The listing builds one solid part. Answer for the finished solid, in the listing's coordinates (mm). A direction names the side the tool comes from. Coordinates: 2 decimals unless noted, no trailing zeros. Order: outer loops, then holes, each group sorted by start corner. A loop starts at its lowest first (then second) coordinate and runs counter-clockwise, first axis right, second up. Notation, with made-up numbers: (49.5, 52) -> (108.5, 52) arc R32 ccw to (108.5, 85) -> close; hole circle Ø4 at (53.25, 10). An arc over 180 degrees is marked (long way). Return JSON: item names as keys, results as strings.
```python
from build123d import *

# Parameters (mm, degrees)
SKETCH1_W           = 50
SKETCH1_H           = 50
BOSS_EXTRUDE1_DEPTH = 25
SHELL1_T            = -2
SKETCH3_W           = 10
SKETCH3_H           = 6
CUT_EXTRUDE1_DEPTH  = 12
SKETCH2_R           = 1.5
CUT_EXTRUDE2_DEPTH  = 44.301270189


with BuildPart() as part:
    # Sketch1 → Boss-Extrude1 (new body)
    with BuildSketch(Plane(origin=(0, 0, 0), x_dir=(1, 0, 0), z_dir=(0, 1, 0))):
        Rectangle(SKETCH1_W, SKETCH1_H)
    extrude(amount=BOSS_EXTRUDE1_DEPTH)

    # Shell1
    shell1_openings = [part.faces().sort_by_distance(p)[0] for p in [
        (0, 0, 0),
    ]]
    offset(amount=SHELL1_T, openings=shell1_openings, kind=Kind.INTERSECTION)

    # Sketch3 → Cut-Extrude1 (cut)
    with BuildSketch(Plane.XY.offset(25)):
        with Locations((-9.833582111, 18.831840126)):
            Rectangle(SKETCH3_W, SKETCH3_H)
    extrude(amount=-CUT_EXTRUDE1_DEPTH, mode=Mode.SUBTRACT)

    # Sketch2 → Cut-Extrude2 (cut, through all)
    with BuildSketch(Plane(origin=(0, 25, 0), x_dir=(1, 0, 0), z_dir=(0, 1, 0))):
        with Locations(Location((15, 0, 0), (0, 0, 270))):
            Circle(SKETCH2_R)
        with Locations(Location((-15, 0, 0), (0, 0, 270))):
            Circle(SKETCH2_R)
        with Locations(Location((-22, 15, 0), (0, 0, 270))):
            Circle(SKETCH2_R)
        with Locations(Location((22, 15, 0), (0, 0, 311.810314896))):
            Circle(SKETCH2_R)
        with Locations(Location((22, -15, 0), (0, 0, 270))):
            Circle(SKETCH2_R)
        with Locations(Location((-22, -15, 0), (0, 0, 228.189685104))):
            Circle(SKETCH2_R)
    extrude(amount=-CUT_EXTRUDE2_DEPTH, mode=Mode.SUBTRACT)


solid = part.part
```
Item 1: Flat-ended cylindrical pins translate along their axes: pin 1 (3.5 mm diameter, centred on x = 15, z = 0, fed in from -Y); pin 2 (2.5 mm diameter, centred on x = 22, z = 15, fed in from -Y). Find the tip coordinate at first contact, or state that the pin passes through.
Answer list:
{"pin 1": "y = 23", "pin 2": "through"}
Item 2: The part is cut by section C-C on y = 5.5. Determine the outline of the cut face in (x, z).
Answer list:
{"outline": "(-25, -25) -> (25, -25) -> (25, 25) -> (-25, 25) -> close; hole (-23, -23) -> (23, -23) -> (23, -16.12) arc R1.5 ccw to (23, -13.88) -> (23, 13.88) arc R1.5 ccw to (23, 16.12) -> (23, 23) -> (-23, 23) -> (-23, 16.12) arc R1.5 ccw to (-23, 13.88) -> (-23, -13.88) arc R1.5 ccw to (-23, -16.12) -> close"}
Item 3: The part is cut by section D-D on x = 22. Determine the outline of the cut face in (y, z), plus the area to 3 significant figures.
Answer list:
{"outline": "(0, -25) -> (25, -25) -> (25, -16.5) -> (23, -16.5) -> (23, -23) -> (0, -23) -> close; (0, 23) -> (23, 23) -> (23, 16.5) -> (25, 16.5) -> (25, 25) -> (0, 25) -> close; (23, -13.5) -> (25, -13.5) -> (25, 13.5) -> (23, 13.5) -> close", "area": "180 mm2"}
Item 4: The part is cut by section B-B on x = 15. Determine the outline of the cut face in (y, z), plus the area to 3 significant figures.
Answer list:
{"outline": "(0, -25) -> (25, -25) -> (25, -1.5) -> (23, -1.5) -> (23, -23) -> (0, -23) -> close; (0, 23) -> (23, 23) -> (23, 1.5) -> (25, 1.5) -> (25, 25) -> (0, 25) -> close", "area": "186 mm2"}
Item 5: Determine the mould class of faces 1 (the flat face through (-10, 21.832, 24)), 2 (the flat face through (0, 23, 0)), 3 (the cylindrical face through (-23.5, 14.41, -14.93)) for opening direction Y: pulls with the +Y half, pulls with the -Y half, needs draft (parallel to the pull), parting line crosses it, or undercut.
Answer list:
{"face 1": "undercut", "face 2": "pulls with the -Y half", "face 3": "needs draft"}
Item 6: Which of the six approach directions +Z, -Z, +X, -X, +Y, -Y give full straight-line access (tool end or side, diameter ignored) to faces 4 (the flat face through (-4.834, 19, 24)), 5 (the cylindrical face through (-23.455, 14.41, 15.363)), 6 (the flat face through (-23, 11, 0))?
Answer list:
{"face 4": "+Z", "face 5": "+Y, -Y", "face 6": "-Y"}
Item 7: Find the intervals of material crossed by probe 1 along Z at (x, y) = (-16.5, 14.5); probe 2 along X at (y, z) = (18, 15), in increasing order.
Answer list:
{"probe 1": "-25 to -23, 23 to 25", "probe 2": "-25 to -23.5, 23.5 to 25"}
Item 8: The part is cut by section A-A on z = 0. Determine the outline of the cut face in (x, y), plus the area to 3 significant figures.
Answer list:
{"outline": "(-25, 0) -> (-23, 0) -> (-23, 23) -> (-16.5, 23) -> (-16.5, 25) -> (-25, 25) -> close; (-13.5, 23) -> (13.5, 23) -> (13.5, 25) -> (-13.5, 25) -> close; (16.5, 23) -> (23, 23) -> (23, 0) -> (25, 0) -> (25, 25) -> (16.5, 25) -> close", "area": "180 mm2"}
